from build123d import *

# Parameters (mm, degrees)
BOSS_EXTRUDE1_DEPTH = 15


with BuildPart() as part:
    # Sketch1 → Boss-Extrude1 (new, symmetric)
    with BuildSketch(Plane.XY):
        with BuildLine():
            Line((-20, 35), (-20, 25))
            Line((-20, 25), (-10, 25))
            ThreePointArc((-10, 25), (0, 15), (10, 25))
            Line((10, 25), (20, 25))
            Line((20, 25), (20, 35))
            Line((20, 35), (30, 35))
            Line((30, 35), (30, 0))
            Line((30, 0), (-30, 0))
            Line((-30, 0), (-30, 35))
            Line((-30, 35), (-20, 35))
        make_face()
    extrude(amount=BOSS_EXTRUDE1_DEPTH, both=True)


solid = part.part
Build history of the part. All positions in model axes, mm. A direction names the side the tool comes from. Give positions to 0.01 mm unless a question says otherwise; leave off trailing zeros. Loops run counter-clockwise (first coordinate to the right, second up) from the corner with the lowest first, then second, coordinate; pieces in that order, holes last. Notation, with made-up numbers: (-1.75, 22.25) -> (32.25, 22.25) arc R19 ccw to (32.25, 53.25) -> close; hole circle Ø2 at (53, -30.5). An arc over 180 degrees is marked (long way). Answer in a Markdown table with one row per item.
Item 1: Slice it at A-A on y = 31.5. Write the cut outline in (x, z), plus the area to 3 significant figures.
Findings below:
| item | result |
|---|---|
| outline | (-30, -15) -> (-20, -15) -> (-20, 15) -> (-30, 15) -> close; (20, -15) -> (30, -15) -> (30, 15) -> (20, 15) -> close |
| area | 600 mm² |
Item 2: Slice it at B-B on z = 5. Write the cut outline in (x, y), plus the area to 3 significant figures.
Findings below:
| item | result |
|---|---|
| outline | (-30, 0) -> (30, 0) -> (30, 35) -> (20, 35) -> (20, 25) -> (10, 25) arc R10 cw to (-10, 25) -> (-20, 25) -> (-20, 35) -> (-30, 35) -> close |
| area | 1,540 mm² |
Item 3: Tool access for faces 5 (the flat face through (-15, 25, 0)), 6 (the flat face through (0, 14, -15)): list every direction of +Z, -Z, +X, -X, +Y, -Y with a clear straight run to the whole face (end or side of a thin tool).
Findings below:
| item | result |
|---|---|
| face 5 | +Z, -Z, +Y |
| face 6 | -Z, +X, -X, +Y, -Y |
Item 4: Probe line 1 along X through (y, z) = (32.5, 14); line 2 along Y through (x, z) = (18.5, -10); line 3 along X through (y, z) = (21, 13). List the from-to ranges inside material, lowest first. Write a range as [from, to].
Findings below:
| item | result |
|---|---|
| line 1 | x = [-30, -20], [20, 30] |
| line 2 | y = [0, 25] |
| line 3 | x = [-30, -9.17], [9.17, 30] |
Item 5: Mould opens along X. For faces 1 (the flat face through (0, 14, 15)), 2 (the flat face through (-20, 30, 0)), 3 (the flat face through (30, 18, 0)), 4 (the flat face through (15, 25, 0)) say: pulls with the +X half, pulls with the -X half, needs draft (parallel to the pull), parting line crosses it, or undercut.
Findings below:
| item | result |
|---|---|
| face 1 | needs draft |
| face 2 | undercut |
| face 3 | pulls with the +X half |
| face 4 | undercut |
Item 6: Slice it at C-C on x = 0. Write the cut outline in (y, z), plus the area to 3 significant figures.
Findings below:
| item | result |
|---|---|
| outline | (0, -15) -> (15, -15) -> (15, 15) -> (0, 15) -> close |
| area | 450 mm² |
Item 7: Flat gauge pin, fed straight in: P1, Ø8, axis at x = 14.5, z = 2, coming from the +Y side. Where does the tip first touch, or does it go through?
Findings below:
| item | result |
|---|---|
| P1 | stops at y = 25 |
Item 8: Slice it at D-D on y = 18. Write the cut outline in (x, z).
Findings below:
| item | result |
|---|---|
| outline | (-30, -15) -> (-7.14, -15) -> (-7.14, 15) -> (-30, 15) -> close; (7.14, -15) -> (30, -15) -> (30, 15) -> (7.14, 15) -> close |
